from build123d import *

# Parameters (mm, degrees)
SKETCH1_W           = 74
SKETCH1_H           = 120
BOSS_EXTRUDE1_DEPTH = 2
SKETCH3_R           = 2.9
CUT_EXTRUDE1_DEPTH  = 71.519500849
FILLET1_R           = 5
SKETCH5_R           = 1.75
CUT_EXTRUDE2_DEPTH  = 71.519500849


with BuildPart() as part:
    # Sketch1 → Boss-Extrude1 (new body)
    with BuildSketch(Plane(origin=(0, 0, 0), x_dir=(1, 0, 0), z_dir=(0, 1, 0))):
        Rectangle(SKETCH1_W, SKETCH1_H)
    extrude(amount=BOSS_EXTRUDE1_DEPTH)

    # Sketch3 → Cut-Extrude1 (cut, through all)
    with BuildSketch(Plane(origin=(0, 2, 0), x_dir=(1, 0, 0), z_dir=(0, 1, 0))):
        with Locations(Location((0, 54, 0), (0, 0, 270))):
            Circle(SKETCH3_R)
        with BuildLine():
            Line((-29, 56.9), (-10, 56.9))
            ThreePointArc((-10, 56.9), (-7.1, 54), (-10, 51.1))
            Line((-10, 51.1), (-29, 51.1))
            ThreePointArc((-29, 51.1), (-31.9, 54), (-29, 56.9))
        make_face()
        with BuildLine():
            Line((10, 56.9), (29, 56.9))
            ThreePointArc((29, 56.9), (31.9, 54), (29, 51.1))
            Line((29, 51.1), (10, 51.1))
            ThreePointArc((10, 51.1), (7.1, 54), (10, 56.9))
        make_face()
    cut_extrude1 = extrude(amount=-CUT_EXTRUDE1_DEPTH, mode=Mode.SUBTRACT)

    # Mirror1: Cut-Extrude1 across plane
    add(cut_extrude1.mirror(Plane.XY), mode=Mode.SUBTRACT)

    # Fillet1
    fillet1_edges = [part.edges().sort_by_distance(p)[0] for p in [
        (37, 1, 60),
        (-37, 1, 60),
        (-37, 1, -60),
        (37, 1, -60),
    ]]
    fillet(fillet1_edges, radius=FILLET1_R)

    # Sketch5 → Cut-Extrude2 (cut, through all)
    with BuildSketch(Plane(origin=(0, 2, 0), x_dir=(1, 0, 0), z_dir=(0, 1, 0))):
        with Locations(Location((-28.25, 35.75, 0), (0, 0, 270))):
            Circle(SKETCH5_R)
        with Locations(Location((28.25, 35.75, 0), (0, 0, 270))):
            Circle(SKETCH5_R)
        with Locations(Location((-28.25, -35.75, 0), (0, 0, 270))):
            Circle(SKETCH5_R)
        with Locations(Location((28.25, -35.75, 0), (0, 0, 270))):
            Circle(SKETCH5_R)
    extrude(amount=-CUT_EXTRUDE2_DEPTH, mode=Mode.SUBTRACT)


solid = part.part
Build history of the part. All positions in model axes, mm. A direction names the side the tool comes from. Round coordinates to 2 decimals unless told otherwise and drop trailing zeros. Write each loop counter-clockwise with the first axis right and the second up, starting at its lowest first coordinate (ties: lowest second). Pieces come first, ordered by that corner, then holes. Notation, with made-up numbers: M 58,-0.5 L 98,-0.5 A17 cw 98,21.5 Z; hole C 49.25,43 d1. An arc over 180 degrees is marked long. Answer as a JSON object with one key per item and string values. Group by question number.
(1) Cut at C-C (y = 1.4). Give the number of separate pieces and of enclosed holes in the cut face, and give its area (3 significant figures).
(2) Flat gauge pin, fed straight in: pin 1 (3 mm diameter, centred on x = -28.25, z = -35.75, fed in from +Y). Where does the tip first touch, or does it go through?
(3) Drill centre lines: L1, parallel to Z at x = 18, y = 1.7; L2, parallel to X at y = 1.1, z = -54; L3, parallel to X at y = 0.8, z = -35.75. Where is each one in solid material? Low to high.
(4) Cut at A-A (x = 20.5). Give the cut face in (y, z).
(5) Mould opens along Z. For faces 3 (the cylindrical face through (35, 1, 59)), 4 (the cylindrical face through (-36, 1, -58)), 5 (the cylindrical face through (-28.92, 1.014, -34.133)), 6 (the cylindrical face through (7.1, 1, 53.9)) say: pulls with the +Z half, pulls with the -Z half, needs draft (parallel to the pull), parting line crosses it, or undercut.
(6) Cut at B-B (z = -35.75). Give the cut face in (x, y), and give its area (3 significant figures).
(7) Which spindle directions (+Z, -Z, +X, -X, +Y, -Y) get a long thin tool onto all of the face, cutting with end or side? Do faces 1 (the cylindrical face through (-36, 1, 58)), 2 (the cylindrical face through (31.9, 1, -54.1)). Say none if no direction does.
Responses:
{
 "1": {"separate pieces": "1", "enclosed holes": "10", "area": "8,220 mm2"},
 "2": {"pin 1": "passes through"},
 "3": {"L1": "z = -60 to -56.9, -51.1 to 51.1, 56.9 to 60", "L2": "x = -37 to -31.9, -7.1 to -2.9, 2.9 to 7.1, 31.9 to 37", "L3": "x = -37 to -30, -26.5 to 26.5, 30 to 37"},
 "4": {"outline": "M 0,-60 L 2,-60 L 2,-56.9 L 0,-56.9 Z; M 0,-51.1 L 2,-51.1 L 2,51.1 L 0,51.1 Z; M 0,56.9 L 2,56.9 L 2,60 L 0,60 Z"},
 "5": {"face 3": "pulls with the +Z half", "face 4": "pulls with the -Z half", "face 5": "undercut", "face 6": "undercut"},
 "6": {"outline": "M -37,0 L -30,0 L -30,2 L -37,2 Z; M -26.5,0 L 26.5,0 L 26.5,2 L -26.5,2 Z; M 30,0 L 37,0 L 37,2 L 30,2 Z", "area": "134 mm2"},
 "7": {"face 1": "+Z, -X, +Y, -Y", "face 2": "+Y, -Y"}
}
